The model under review builds one solid part; all positions refer to its coordinate system, in mm. Face numbers are marked on the shaded views. A direction names the side the tool comes from. Coordinates: 2 decimals unless noted, no trailing zeros. Order: outer loops, then holes, each group sorted by start corner. A loop starts at its lowest first (then second) coordinate and runs counter-clockwise, first axis right, second up. Notation, with made-up numbers: M -6.5,85 L 27.5,85 A16 ccw 27.5,106 Z; hole C 62.25,-29 d5. An arc over 180 degrees is marked long. Write each question's results on one line, items separated by ' | '.
from build123d import *

# Parameters (mm, degrees)
F2_R = 10
F3_R = 5


with BuildPart() as f1:
    # F0 (on Front) → F1 (revolve)
    with BuildSketch(Plane.XZ):
        Polygon((0, 90), (0, 0), (13, 0), (11.11462, 1.88538), (3, 6.2), (3, 85), (1.5, 85), (1.5, 90), align=None)
    revolve(axis=Axis((0, 0, 45), (0, 0, -1)))

    # F2
    f2_edges = [f1.edges().sort_by_distance(p)[0] for p in [
        (-3, 0, 6.2),
    ]]
    fillet(f2_edges, radius=F2_R)

    # F3
    f3_edges = [f1.edges().sort_by_distance(p)[0] for p in [
        (-11.11462, 0, 1.88538),
    ]]
    fillet(f3_edges, radius=F3_R)


solid = f1.part
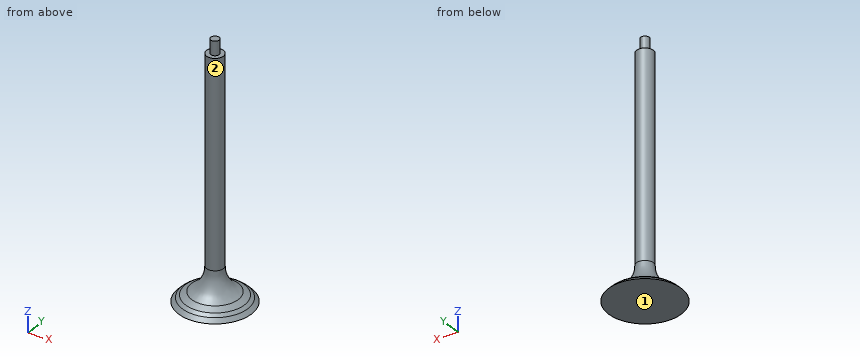
1) Take a section at A-A on z = 72.5. State the section outline as (x, y) points, plus the area to 3 significant figures.
Solutions:
outline: C 0,0 d6 | area: 28.3 mm2
2) For the marked faces 1 and 2, list the 3-axis set-ups (+Z, -Z, +X, -X, +Y, -Y) from which the entire face can be reached by the end or side of a thin tool; tool diameter is ignored.
Solutions:
face 1: -Z, +X, -X, +Y, -Y | face 2: +Z
3) For pin 1 (1 mm diameter, centred on x = -0.5, y = 9, fed in from -Z); pin 2 (8 mm diameter, centred on x = -2.5, z = 48.5, fed in from +Y); pin 3 (12 mm diameter, centred on x = 10, y = 4.5, fed in from +Z); pin 4 (1 mm diameter, centred on x = 2.5, y = 3.5, fed in from +Z), all flat-tipped, find the tip position at first contact; note any pin that passes through.
Solutions:
pin 1: z = 0 | pin 2: y = 3 | pin 3: z = 6.25 | pin 4: z = 8.29
4) To check wall thickness, follow line 1 along Y through (x, z) = (-2.5, 20); line 2 along Z through (x, y) = (-6, 9); line 3 along X through (y, z) = (-2.5, 7). State the ranges of each line that lie inside material, in increasing order.
Solutions:
line 1: -1.66 to 1.66 | line 2: 0 to 2.02 | line 3: -3.7 to 3.7
